from build123d import *

# Parameters (mm, degrees)
SKETCH1_R           = 15
BOSS_EXTRUDE1_DEPTH = 15
CUT_EXTRUDE1_DEPTH  = 16
CIRPATTERN1_COUNT   = 16
SKETCH3_R           = 2.5
CUT_EXTRUDE2_DEPTH  = 16


with BuildPart() as part:
    # Sketch1 → Boss-Extrude1 (new body)
    with BuildSketch(Plane.XY):
        Circle(SKETCH1_R)
    extrude(amount=BOSS_EXTRUDE1_DEPTH)

    # Sketch2 → Cut-Extrude1 (cut, through all)
    with BuildSketch(Plane.XY.offset(15)):
        with BuildLine():
            ThreePointArc((-1, 10.95445115), (0, 11), (1, 10.95445115))
            ThreePointArc((1, 10.95445115), (1.384034944, 13.063153145), (2.7, 14.754999153))
            ThreePointArc((2.7, 14.754999153), (0, 15), (-2.7, 14.754999153))
            ThreePointArc((-2.7, 14.754999153), (-1.384034944, 13.063153145), (-1, 10.95445115))
        make_face()
    cut_extrude1 = extrude(amount=-CUT_EXTRUDE1_DEPTH, mode=Mode.SUBTRACT)

    # CirPattern1: Cut-Extrude1 ×16 about axis
    cirpattern1_axis = Axis((0, 0, 0), (0, 0, 1))
    for i in range(1, CIRPATTERN1_COUNT):
        add(cut_extrude1.rotate(cirpattern1_axis, i * 360 / CIRPATTERN1_COUNT), mode=Mode.SUBTRACT)

    # Sketch3 → Cut-Extrude2 (cut, through all)
    with BuildSketch(Plane.XY.offset(15)):
        Circle(SKETCH3_R)
    extrude(amount=-CUT_EXTRUDE2_DEPTH, mode=Mode.SUBTRACT)


solid = part.part
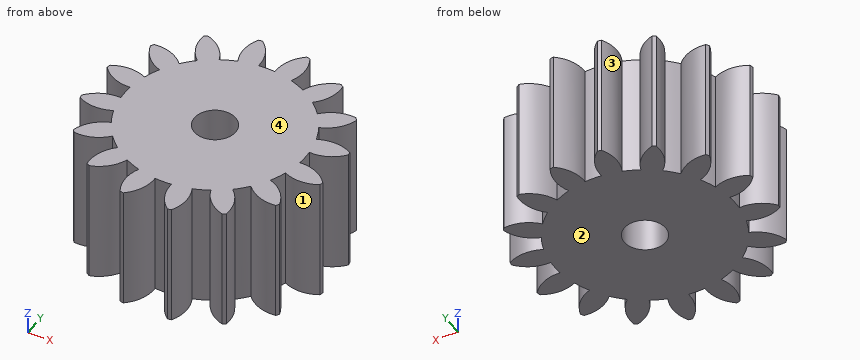
Part model, mm, in its own coordinate system. Face numbers are marked on the shaded views. A direction names the side the tool comes from. Coordinates: 2 decimals unless noted, no trailing zeros. Order: outer loops, then holes, each group sorted by start corner. A loop starts at its lowest first (then second) coordinate and runs counter-clockwise, first axis right, second up.
(1) Probe L1, parallel to Y at x = 0, z = 6; L2, parallel to X at y = 12, z = 12; L3, parallel to X at y = -11.5, z = 5.75. List the from-to ranges inside material, lowest first.
Check sheet entries:
L1: y = -11 to -2.5, 2.5 to 11
L2: x = -8.55 to -6.85, -3.7 to -1.06, 1.06 to 3.7, 6.85 to 8.55
L3: x = -8.54 to -6.24, -3.62 to -1, 1 to 3.62, 6.24 to 8.54
(2) Pin check, flat tips, straight feed: pin 1 Ø4 at (x, y) = (6, -1.5) entering from -Z; pin 2 Ø6 at (y, z) = (2, 7.5) entering from +X (3 decimals); pin 3 Ø1.5 at (x, z) = (-1, 8.5) entering from -Y; pin 4 Ø2 at (y, z) = (-10.5, 13.5) entering from +X. Stop position of each tip, or through.
Check sheet entries:
pin 1: stops at z = 0
pin 2: stops at x = 14.755
pin 3: stops at y = -13.73
pin 4: stops at x = 8.54
(3) Tool access for the marked faces 1 and 2: list every direction of +Z, -Z, +X, -X, +Y, -Y with a clear straight run to the whole face (end or side of a thin tool).
Check sheet entries:
face 1: +Z, -Z
face 2: -Z, +X, -X, +Y, -Y
(4) Slice it at A-A, the plane x = 0. Write the cut outline in (y, z).
Check sheet entries:
outline: (-11, 0) - (-2.5, 0) - (-2.5, 15) - (-11, 15) - close; (2.5, 0) - (11, 0) - (11, 15) - (2.5, 15) - close
(5) Pull direction X, two halves, no side cores. Call the marked faces 3 and 4: pulls with the +X half, pulls with the -X half, needs draft (parallel to the pull), parting line crosses it, or undercut.
Check sheet entries:
face 3: undercut
face 4: needs draft
